from build123d import *

# Parameters (mm, degrees)
BASE_FLANGE1_DEPTH            = 9.525
EDGE_FLANGE1_STRIP_W          = 50.8508
EDGE_FLANGE1_STRIP_H          = 9.525
EDGE_FLANGE1_STRIP_CUT_DEPTH  = 254
EDGE_FLANGE1_RELIEF_W         = 55.6133
EDGE_FLANGE1_RELIEF_H         = 4.7625
EDGE_FLANGE1_RELIEF_CUT_DEPTH = 9.525
EDGE_FLANGE1_DEPTH            = 254


# Sheet-metal steps are written as plain solids
with BuildPart() as part:
    # Sketch1 → Base-Flange1 (new body)
    with BuildSketch(Plane(origin=(0, 0, 0), x_dir=(1, 0, 0), z_dir=(0, 1, 0))):
        Polygon((304.8, 50.8), (304.8, 203.2), (-152.4, 203.2), (-304.8, 50.8), (-304.8, -50.8), (-152.4, -254), (0, -254), (304.8, -50.8), align=None)
    extrude(amount=-BASE_FLANGE1_DEPTH)

    # Edge-Flange1 strip (across the edge) → Edge-Flange1 strip cut (cut)
    with BuildSketch(Plane(origin=(304.8, -9.525, -203.2), x_dir=(-1, 0, 0), z_dir=(0, 0, 1))):
        with Locations((-19.05, -4.7625)):
            Rectangle(EDGE_FLANGE1_STRIP_W, EDGE_FLANGE1_STRIP_H)
    extrude(amount=EDGE_FLANGE1_STRIP_CUT_DEPTH, mode=Mode.SUBTRACT)

    # Edge-Flange1 relief (on the sheet) → Edge-Flange1 relief cut (cut)
    with BuildSketch(Plane(origin=(298.4246, -9.525, -203.2), x_dir=(-1, 0, 0), z_dir=(0, -1, 0))):
        with Locations((-23.04415, -256.38125)):
            Rectangle(EDGE_FLANGE1_RELIEF_W, EDGE_FLANGE1_RELIEF_H)
    extrude(amount=-EDGE_FLANGE1_RELIEF_CUT_DEPTH, mode=Mode.SUBTRACT)

    # Edge-Flange1 section (across the edge) → Edge-Flange1 (add)
    with BuildSketch(Plane(origin=(304.8, -9.525, -203.2), x_dir=(-1, 0, 0), z_dir=(0, 0, 1))):
        with BuildLine():
            Line((-9.525, 6.3754), (-9.525, 152.4))
            Line((-9.525, 152.4), (0, 152.4))
            Line((0, 152.4), (0, 6.3754))
            ThreePointArc((0, 6.3754), (1.867311427, 1.867311427), (6.3754, 0))
            Line((6.3754, 0), (6.3754, -9.525))
            ThreePointArc((6.3754, -9.525), (-4.867880664, -4.867880664), (-9.525, 6.3754))
        make_face()
    extrude(amount=EDGE_FLANGE1_DEPTH)


solid = part.part
For this review, take the finished solid that the model builds, in its own axes (mm). A direction names the side the tool comes from. Round coordinates to 2 decimals unless told otherwise and drop trailing zeros. Order: outer loops, then holes, each group sorted by start corner. A loop starts at its lowest first (then second) coordinate and runs counter-clockwise, first axis right, second up. Notation, with made-up numbers: (47.5, 29.25) -> (100.5, 29.25) arc R14 cw to (100.5, 37.25) -> close; hole circle Ø9 at (54, 33). An arc over 180 degrees is marked (long way). Write item = value, one per line. Start each with the question number.
1) Take a section at B-B on y = -140. State the section outline as (x, z) points (3 decimals).
2) To check wall thickness, follow line 1 (Y direction, x = -28.5, z = -40.5) (3 decimals); line 2 (X direction, y = -47.5, z = 24) (3 decimals). State the ranges of each line that lie inside material, in increasing order. Write a range as from..to.
3) The part is to be moulded in two halves that separate along Y. For faces 1 (the face through (-229.667, -4.696, 150.978)), 2 (the face through (-7, 0, 22)), 3 (the face through (-7, -9.525, 22)), say which applies: +Y half, -Y half, draft (parallel to the pull), parting line (faces both ways), or undercut.
4) Tool access review of faces 4 (the face through (304.8, -90, -78)), 5 (the face through (80, -9, -203.2)): name each direction out of +Z, -Z, +X, -X, +Y, -Y from which nothing blocks a thin tool from reaching the whole face with its end or side.
5) Insertion check: pin 1 (22.5 mm diameter, centred on x = 306, y = -104, fed in from +Z); pin 2 (8 mm diameter, centred on x = -47.5, z = 47.5, fed in from -Y) (3 decimals); pin 3 (4 mm diameter, centred on y = -4.5, z = 53, fed in from +X). Each pin has a flat end and moves straight along its axis. Give the tip position at first contact, or say it passes through.
6) Take a section at C-C on x = -123.5. State the section outline as (y, z) points (3 decimals).
7) Take a section at A-A on z = -39.5. State the section outline as (x, y) points (3 decimals), plus the area to 3 significant figures.
8) Take a section at D-D on z = -137.5. State the section outline as (x, y) points (3 decimals), plus the area to 3 significant figures.
Verdict:
q1.outline = (304.8, -203.2) -> (314.325, -203.2) -> (314.325, 50.8) -> (304.8, 50.8) -> close
q2.line_1 = -9.525..0
q2.line_2 = 304.8..314.325
q3.face_1 = draft
q3.face_2 = +Y half
q3.face_3 = -Y half
q4.face_4 = +Z, -Z, -X, -Y
q4.face_5 = -Z, +X, -X, +Y, -Y
q5.pin_1 = 50.8
q5.pin_2 = -9.525
q5.pin_3 = 293.66
q6.outline = (-9.525, -203.2) -> (0, -203.2) -> (0, 254) -> (-9.525, 254) -> close
q7.outline = (-304.8, -9.525) -> (298.425, -9.525) arc R6.375 cw to (304.8, -15.9) -> (304.8, -161.925) -> (314.325, -161.925) -> (314.325, -15.9) arc R15.9 ccw to (298.425, 0) -> (-304.8, 0) -> close
q7.area = 7,300 mm2
q8.outline = (-218.1, -9.525) -> (298.425, -9.525) arc R6.375 cw to (304.8, -15.9) -> (304.8, -161.925) -> (314.325, -161.925) -> (314.325, -15.9) arc R15.9 ccw to (298.425, 0) -> (-218.1, 0) -> close
q8.area = 6,480 mm2
